Drawing for the job (mm, zero at the part's lowest x, y, z). A direction names the side the tool comes from. Give positions to 0.01 mm unless a question says otherwise; leave off trailing zeros. Loops run counter-clockwise (first coordinate to the right, second up) from the corner with the lowest first, then second, coordinate; pieces in that order, holes last. Notation, with made-up numbers: (19, 59.5) -> (35, 59.5) arc R11 ccw to (35, 76.5) -> close; hole circle Ø3 at (-36, 85.25). An arc over 180 degrees is marked (long way). Answer in a Markdown table with one row per item. Add a question column.
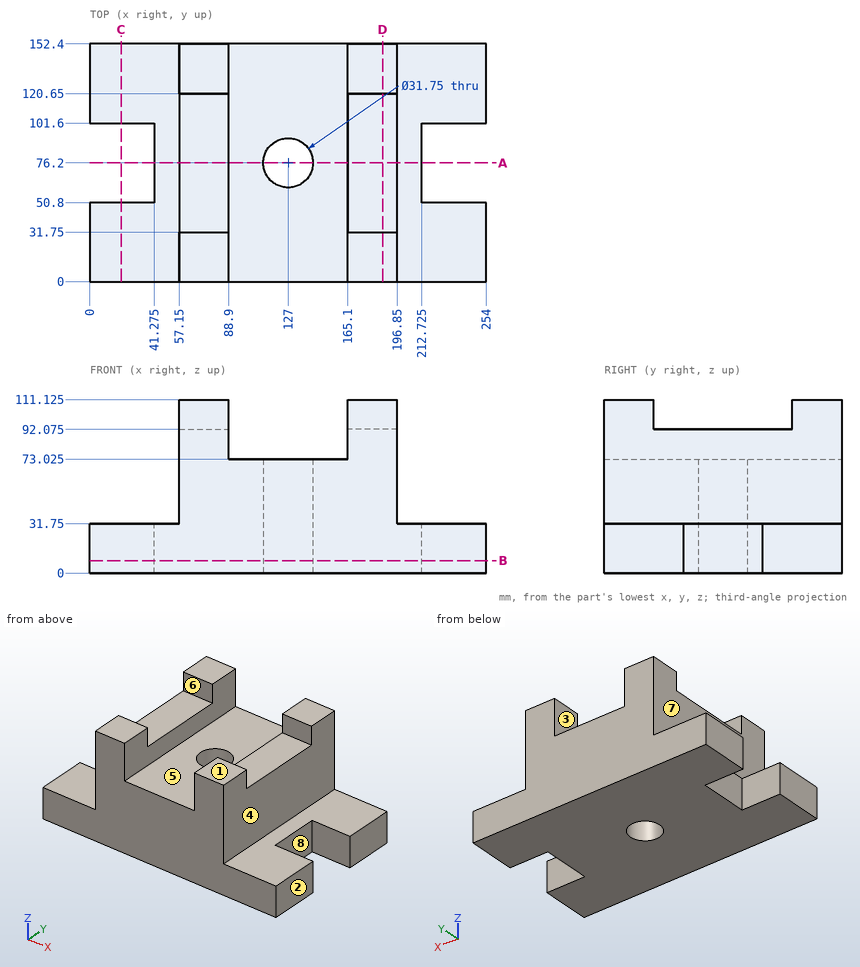
(1) Saw through at B-B, the plane z = 8. List the corners of the cut face in (x, y) (3 decimals), then the cut area to 3 significant figures.
(2) 3-axis set-ups, long thin cutter, end or side, ignore diameter. For the marked faces 4, 5, 6, 7 and 8: which of +Z, -Z, +X, -X, +Y, -Y reach the whole face in a straight line?
(3) Flat gauge pins, fed straight in: pin 1 Ø1 at (x, y) = (157, 67.5) entering from +Z (3 decimals); pin 2 Ø3 at (y, z) = (119, 90.5) entering from +X; pin 3 Ø8 at (y, z) = (91.5, 15) entering from -X (3 decimals). Where does each tip first touch, or does it go through?
(4) Saw through at D-D, the plane x = 187.5. List the corners of the cut face in (y, z) (3 decimals), then the cut area to 3 significant figures.
(5) Two-plate mould, pull along X, no slides. Class the marked faces 1, 2 and 3: released by +X, released by -X, zero draft, split by the parting line, or undercut.
(6) Saw through at A-A, the plane y = 76.2. List the corners of the cut face in (x, z) (3 decimals).
(7) Wall check: line 1 along Y through (x, z) = (127, 26) (3 decimals); line 2 along Y through (x, z) = (77.5, 99); line 3 along X through (y, z) = (12.5, 93). Give the ranges that are in metal, low to high. Write a range as from..to.
(8) Saw through at C-C, the plane x = 20. List the corners of the cut face in (y, z), then the cut area to 3 significant figures.
Worked answers:
| question | item | result |
|---|---|---|
| 1 | outline | (0, 0) -> (254, 0) -> (254, 50.8) -> (212.725, 50.8) -> (212.725, 101.6) -> (254, 101.6) -> (254, 152.4) -> (0, 152.4) -> (0, 101.6) -> (41.275, 101.6) -> (41.275, 50.8) -> (0, 50.8) -> close; hole circle Ø31.75 at (127, 76.2) |
| 1 | area | 33,700 mm^2 |
| 2 | face 4 | +Z, +X, +Y, -Y |
| 2 | face 5 | +Z, +Y, -Y |
| 2 | face 6 | +Z, +X, -X |
| 2 | face 7 | +Z, -X, +Y, -Y |
| 2 | face 8 | +Z, -Z, +X |
| 3 | pin 1 | z = 73.025 |
| 3 | pin 2 | x = 196.85 |
| 3 | pin 3 | x = 41.275 |
| 4 | outline | (0, 0) -> (152.4, 0) -> (152.4, 111.125) -> (120.65, 111.125) -> (120.65, 92.075) -> (31.75, 92.075) -> (31.75, 111.125) -> (0, 111.125) -> close |
| 4 | area | 15,200 mm^2 |
| 5 | face 1 | zero draft |
| 5 | face 2 | released by +X |
| 5 | face 3 | undercut |
| 6 | outline | (41.275, 0) -> (111.125, 0) -> (111.125, 73.025) -> (88.9, 73.025) -> (88.9, 92.075) -> (57.15, 92.075) -> (57.15, 31.75) -> (41.275, 31.75) -> close; (142.875, 0) -> (212.725, 0) -> (212.725, 31.75) -> (196.85, 31.75) -> (196.85, 92.075) -> (165.1, 92.075) -> (165.1, 73.025) -> (142.875, 73.025) -> close |
| 7 | line 1 | 0..60.325, 92.075..152.4 |
| 7 | line 2 | 0..31.75, 120.65..152.4 |
| 7 | line 3 | 57.15..88.9, 165.1..196.85 |
| 8 | outline | (0, 0) -> (50.8, 0) -> (50.8, 31.75) -> (0, 31.75) -> close; (101.6, 0) -> (152.4, 0) -> (152.4, 31.75) -> (101.6, 31.75) -> close |
| 8 | area | 3,230 mm^2 |
